```python
from build123d import *

# Parameters (mm, degrees)
EXTRUDE_1_DEPTH          = 124
SKETCH_2_W               = 160
SKETCH_2_H               = 55.63
EXTRUDE_2_DEPTH          = 6
CUT_EXTRUDE_1_DEPTH      = 186.458073159
CUT_EXTRUDE_1_DEPTH_BACK = 186.458073159
SHELL_START              = -78
SHELL_1_OUTLINE_W        = 53.63
SHELL_1_OUTLINE_H        = 126
SHELL_1_DEPTH            = 156
SHELL_START_2            = -38
SHELL_1_2_DEPTH          = 76
SKETCH_6_W               = 156
SKETCH_6_H               = 53.63
CUT_EXTRUDE_2_DEPTH      = 3
EXTRUDE_3_DEPTH          = 2
SKETCH_8_R               = 23.405642618
CUT_EXTRUDE_3_DEPTH      = 231.346358066
EXTRUDE_4_DEPTH          = 2
EXTRUDE_START            = -2
EXTRUDE_5_DEPTH          = 2
SKETCH_11_R              = 3
CUT_EXTRUDE_4_DEPTH      = 248.192749183


# Read off the part's stored shape, not the designer's step: 抽壳1
with BuildPart() as part:
    # 草图1 → 凸台-拉伸1 (new body)
    with BuildSketch(Plane.XY):
        Polygon((-80, 0), (-40, 0), (-40, -48), (40, -48), (40, 0), (80, 0), (80, 55.63), (-80, 55.63), align=None)
    extrude(amount=EXTRUDE_1_DEPTH)

    # 草图2 → 凸台-拉伸2 (add)
    with BuildSketch(Plane.XY.offset(124)):
        with Locations((0, 27.815)):
            Rectangle(SKETCH_2_W, SKETCH_2_H)
    extrude(amount=EXTRUDE_2_DEPTH)

    # 草图4 → 切除-拉伸1 (cut, two sides: drawn at the far end of the back side and taken through both)
    with BuildSketch(Plane.ZY.offset(40).offset(-CUT_EXTRUDE_1_DEPTH_BACK)):
        with BuildLine():
            Line((124, 0), (97.256578086, -43.258479388))
            ThreePointArc((97.256578086, -43.258479388), (93.619837537, -46.734551903), (88.750792142, -48))
            Line((88.750792142, -48), (88.750792142, -53.726448165))
            Line((88.750792142, -53.726448165), (126.100983763, -53.726448165))
            Line((126.100983763, -53.726448165), (126.100983763, 0))
            Line((126.100983763, 0), (124, 0))
        make_face()
    extrude(amount=CUT_EXTRUDE_1_DEPTH + CUT_EXTRUDE_1_DEPTH_BACK, mode=Mode.SUBTRACT)

    # 抽壳1 outline → 抽壳1 (cut)
    with BuildSketch(Plane.YZ.offset(SHELL_START)):
        with Locations((28.815, 65)):
            Rectangle(SHELL_1_OUTLINE_W, SHELL_1_OUTLINE_H)
    extrude(amount=SHELL_1_DEPTH, mode=Mode.SUBTRACT)

    # Shell 1 2 outline → Shell 1 2 (cut)
    with BuildSketch(Plane.YZ.offset(SHELL_START_2)):
        with BuildLine():
            Line((-46, 88.750792142), (-46, 2))
            Line((-46, 2), (2, 2))
            Line((2, 2), (2, 122.885106998))
            Line((2, 122.885106998), (-42.20678351, 95.555420897))
            ThreePointArc((-42.20678351, 95.555420897), (-44.987641522, 92.646028458), (-46, 88.750792142))
        make_face()
    extrude(amount=SHELL_1_2_DEPTH, mode=Mode.SUBTRACT)

    # 草图6 → 切除-拉伸2 (cut)
    with BuildSketch(Plane(origin=(0, 0, 128), x_dir=(-1, 0, 0), z_dir=(0, 0, -1))):
        with Locations((0, 28.815)):
            Rectangle(SKETCH_6_W, SKETCH_6_H)
    extrude(amount=-CUT_EXTRUDE_2_DEPTH, mode=Mode.SUBTRACT)

    # 草图7 → 凸台-拉伸3 (add)
    with BuildSketch(Plane.ZY.offset(80)):
        Polygon((130, 55.63), (156.092113107, 55.63), (156.092113107, 29.820089386), (130, 0), align=None)
    extrude(amount=-EXTRUDE_3_DEPTH)

    # 草图8 → 切除-拉伸3 (cut, through all)
    with BuildSketch(Plane.ZY.offset(80)):
        with Locations((163.334420687, 11.150000051)):
            Circle(SKETCH_8_R)
    extrude(amount=-CUT_EXTRUDE_3_DEPTH, mode=Mode.SUBTRACT)

    # 草图9 → 凸台-拉伸4 (add)
    with BuildSketch(Plane.ZY.offset(80)):
        Polygon((156.092113107, 33.406978446), (179.938761178, 33.406978446), (180.026549011, 55.62973882), (156.092113107, 55.63), align=None)
    extrude(amount=-EXTRUDE_4_DEPTH)

    # 草图10 → 凸台-拉伸5 (add)
    with BuildSketch(Plane(origin=(80, 0, 0), x_dir=(0, 0, -1), z_dir=(1, 0, 0)).offset(EXTRUDE_START)):
        with BuildLine():
            Line((-130, 55.63), (-180.026549011, 55.62973882))
            Line((-180.026549011, 55.62973882), (-179.938761178, 33.406978446))
            Line((-179.938761178, 33.406978446), (-156.092113107, 33.406978446))
            ThreePointArc((-156.092113107, 33.406978446), (-144.454345373, 24.983541264), (-139.929618433, 11.348337638))
            Line((-139.929618433, 11.348337638), (-130, 0))
            Line((-130, 0), (-130, 55.63))
        make_face()
    extrude(amount=EXTRUDE_5_DEPTH)

    # 草图11 → 切除-拉伸4 (cut, through all)
    with BuildSketch(Plane(origin=(80, 0, 0), x_dir=(0, 0, -1), z_dir=(1, 0, 0))):
        with Locations((-168.015437143, 42.878856115)):
            Circle(SKETCH_11_R)
    extrude(amount=-CUT_EXTRUDE_4_DEPTH, mode=Mode.SUBTRACT)


solid = part.part
```
Model file for the job. Use its own axes, mm. A direction names the side the tool comes from. Give positions to 0.01 mm unless a question says otherwise; leave off trailing zeros. Write each loop counter-clockwise with the first axis right and the second up, starting at its lowest first coordinate (ties: lowest second). Pieces come first, ordered by that corner, then holes. Notation, with made-up numbers: (-10.75, -28) - (33.25, -28) arc R25 ccw to (33.25, -15) - close; hole circle Ø4 at (58, -37). An arc over 180 degrees is marked (long way). One line per question, with ' | ' between items. Start each with the question number.
(1) 3-axis set-ups, long thin cutter, end or side, ignore diameter. For faces 5 (the face through (-1, -48, 44)), 6 (the face through (53, 2, 65)), 7 (the face through (-79.014, 25.148, 144.576)), 8 (the face through (-40, -24, 61)), 9 (the face through (-0.532, -44.96, 92.696)): which of +Z, -Z, +X, -X, +Y, -Y reach the whole face in a straight line?
(2) Slice it at B-B on y = -31.5. Write the cut outline in (x, z).
(3) Slice it at C-C on x = 26. Write the cut outline in (y, z), plus the area to 3 significant figures.
(4) Wall check: line 1 along X through (y, z) = (-12.5, 45.5); line 2 along X through (y, z) = (14.5, 130.5); line 3 along Z through (x, y) = (3.5, 48.5). Give the ranges that are in metal, low to high. Write a range as from..to.
(5) Slice it at D-D on z = 145. Write the cut outline in (x, y).
(6) Two-plate mould, pull along X, no slides. Class faces 1 (the face through (-79.01, 5.75, 135.03)), 2 (the face through (78, 28, 92)), 3 (the face through (-1, 15, 2)), 4 (the face through (-80, 28, 69)): +X half, -X half, draft (parallel to the pull), parting line (faces both ways), or undercut.
(7) Pin check, flat tips, straight feed: P1, Ø12, axis at x = -55.5, z = 45.5, coming from the -Y side; P2, Ø24, axis at y = -35.5, z = 36, coming from the -X side; P3, Ø0.6, axis at x = 79, z = 168, coming from the -Y side; P4, Ø3.5, axis at y = 42.88, z = 168.02, coming from the +X side. Stop position of each tip, or through.
(8) Slice it at A-A on z = 61. Write the cut outline in (x, y).
Results below:
1) face 5: +Z, -Z, +X, -X, -Y | face 6: +Z, +Y | face 7: +Z, +X, -X, -Y | face 8: +Z, -Z, -X, -Y | face 9: +Y
2) outline: (-40, 0) - (40, 0) - (40, 104.53) - (-40, 104.53) - close; hole (-38, 2) - (38, 2) - (38, 102.17) - (-38, 102.17) - close
3) outline: (-48, 0) - (55.63, 0) - (55.63, 2) - (-46, 2) - (-46, 88.75) arc R8 cw to (-42.21, 95.56) - (2, 122.89) - (2, 130) - (0, 130) - (0, 124) - (-43.26, 97.26) arc R10 ccw to (-48, 88.75) - close | area: 515 mm^2
4) line 1: -40..-38, 38..40 | line 2: -80..-78, 78..80 | line 3: 0..2
5) outline: (-80, 25.7) - (-78, 25.7) - (-78, 55.63) - (-80, 55.63) - close; (78, 25.7) - (80, 25.7) - (80, 55.63) - (78, 55.63) - close
6) face 1: draft | face 2: undercut | face 3: undercut | face 4: -X half
7) P1: y = 0 | P2: x = -40 | P3: y = 33.41 | P4: through
8) outline: (-80, 0) - (-40, 0) - (-40, -48) - (40, -48) - (40, 0) - (80, 0) - (80, 55.63) - (78, 55.63) - (78, 2) - (38, 2) - (38, -46) - (-38, -46) - (-38, 2) - (-78, 2) - (-78, 55.63) - (-80, 55.63) - close
